Build history of the part. All positions in model axes, mm. A direction names the side the tool comes from. Round coordinates to 2 decimals unless told otherwise and drop trailing zeros. Write each loop counter-clockwise with the first axis right and the second up, starting at its lowest first coordinate (ties: lowest second). Pieces come first, ordered by that corner, then holes.
from build123d import *
from OCP.BRepFilletAPI import BRepFilletAPI_MakeChamfer

# Parameters (mm, degrees)
SKETCH1_W                = 15.2
SKETCH1_H                = 8.8
BOSS_EXTRUDE1_DEPTH      = 9
SKETCH3_W                = 13
SKETCH3_H                = 6.4
CUT_EXTRUDE1_DEPTH       = 8
SKETCH4_W                = 4.5
SKETCH4_H                = 1.2
CUT_EXTRUDE2_DEPTH       = 7
SKETCH5_W                = 3
SKETCH5_H                = 7
CUT_EXTRUDE3_DEPTH       = 1.1
SKETCH6_W                = 3
SKETCH6_H                = 7
CUT_EXTRUDE4_DEPTH       = 1.1
BOSS_EXTRUDE2_DEPTH      = 7.5
BOSS_EXTRUDE2_DEPTH_BACK = 4
SKETCH7_W                = 1
SKETCH7_H                = 1
CHAMFER1_SIZE            = 0.7
CHAMFER1_SIZE2           = 0.254779164
CHAMFER2_SIZE            = 0.5


with BuildPart() as part:
    # Sketch1 → Boss-Extrude1 (new body)
    with BuildSketch(Plane(origin=(0, 0, 0), x_dir=(1, 0, 0), z_dir=(0, 1, 0))):
        with Locations((7.6, 4.4)):
            Rectangle(SKETCH1_W, SKETCH1_H)
    extrude(amount=BOSS_EXTRUDE1_DEPTH)

    # Sketch3 → Cut-Extrude1 (cut)
    with BuildSketch(Plane(origin=(0, 9, 0), x_dir=(1, 0, 0), z_dir=(0, 1, 0))):
        with Locations((7.6, 4.4)):
            Rectangle(SKETCH3_W, SKETCH3_H)
    extrude(amount=-CUT_EXTRUDE1_DEPTH, mode=Mode.SUBTRACT)

    # Sketch4 → Cut-Extrude2 (cut)
    with BuildSketch(Plane(origin=(0, 9, 0), x_dir=(1, 0, 0), z_dir=(0, 1, 0))):
        with Locations((7.6, 0.6)):
            Rectangle(SKETCH4_W, SKETCH4_H)
    extrude(amount=-CUT_EXTRUDE2_DEPTH, mode=Mode.SUBTRACT)

    # Sketch5 → Cut-Extrude3 (cut)
    with BuildSketch(Plane.ZY):
        with Locations((-4.4, 3.5)):
            Rectangle(SKETCH5_W, SKETCH5_H)
    extrude(amount=-CUT_EXTRUDE3_DEPTH, mode=Mode.SUBTRACT)

    # Sketch6 → Cut-Extrude4 (cut)
    with BuildSketch(Plane(origin=(15.2, 0, 0), x_dir=(0, 0, -1), z_dir=(1, 0, 0))):
        with Locations((4.4, 3.5)):
            Rectangle(SKETCH6_W, SKETCH6_H)
    extrude(amount=-CUT_EXTRUDE4_DEPTH, mode=Mode.SUBTRACT)

    # Sketch7 → Boss-Extrude2 (add, two sides: drawn at the far end of the back side and taken through both)
    with BuildSketch(Plane(origin=(0, 1, 0), x_dir=(1, 0, 0), z_dir=(0, 1, 0)).offset(-BOSS_EXTRUDE2_DEPTH_BACK)):
        with Locations((7.6, 5.67)):
            Rectangle(SKETCH7_W, SKETCH7_H)
        with Locations((5.06, 5.67)):
            Rectangle(SKETCH7_W, SKETCH7_H)
        with Locations((10.14, 5.67)):
            Rectangle(SKETCH7_W, SKETCH7_H)
        with Locations((7.6, 3.13)):
            Rectangle(SKETCH7_W, SKETCH7_H)
        with Locations((10.14, 3.13)):
            Rectangle(SKETCH7_W, SKETCH7_H)
        with Locations((5.06, 3.13)):
            Rectangle(SKETCH7_W, SKETCH7_H)
    extrude(amount=BOSS_EXTRUDE2_DEPTH + BOSS_EXTRUDE2_DEPTH_BACK)

    # Chamfer1: one chamfer whose edges measure the first distance from different faces: ONE call of the kernel's chamfer builder (chamfer() names one face for all edges)
    chamfer1_edges_1 = [part.edges().sort_by_distance(p)[0] for p in [
        (7.1, 8.5, -5.67),
    ]]
    chamfer1_side_1 = [part.faces().sort_by_distance(p)[0] for p in [
        (7.1, 4.75, -5.67),
    ]]
    chamfer1_edges_2 = [part.edges().sort_by_distance(p)[0] for p in [
        (7.6, 8.5, -5.17),
    ]]
    chamfer1_side_2 = [part.faces().sort_by_distance(p)[0] for p in [
        (7.6, 4.75, -5.17),
    ]]
    chamfer1_edges_3 = [part.edges().sort_by_distance(p)[0] for p in [
        (8.1, 8.5, -5.67),
    ]]
    chamfer1_side_3 = [part.faces().sort_by_distance(p)[0] for p in [
        (8.1, 4.75, -5.67),
    ]]
    chamfer1_edges_4 = [part.edges().sort_by_distance(p)[0] for p in [
        (7.6, 8.5, -6.17),
    ]]
    chamfer1_side_4 = [part.faces().sort_by_distance(p)[0] for p in [
        (7.6, 4.75, -6.17),
    ]]
    chamfer1_edges_5 = [part.edges().sort_by_distance(p)[0] for p in [
        (9.64, 8.5, -5.67),
    ]]
    chamfer1_side_5 = [part.faces().sort_by_distance(p)[0] for p in [
        (9.64, 4.75, -5.67),
    ]]
    chamfer1_edges_6 = [part.edges().sort_by_distance(p)[0] for p in [
        (10.14, 8.5, -5.17),
    ]]
    chamfer1_side_6 = [part.faces().sort_by_distance(p)[0] for p in [
        (10.14, 4.75, -5.17),
    ]]
    chamfer1_edges_7 = [part.edges().sort_by_distance(p)[0] for p in [
        (10.64, 8.5, -5.67),
    ]]
    chamfer1_side_7 = [part.faces().sort_by_distance(p)[0] for p in [
        (10.64, 4.75, -5.67),
    ]]
    chamfer1_edges_8 = [part.edges().sort_by_distance(p)[0] for p in [
        (10.14, 8.5, -6.17),
    ]]
    chamfer1_side_8 = [part.faces().sort_by_distance(p)[0] for p in [
        (10.14, 4.75, -6.17),
    ]]
    chamfer1_edges_9 = [part.edges().sort_by_distance(p)[0] for p in [
        (7.1, 8.5, -3.13),
    ]]
    chamfer1_side_9 = [part.faces().sort_by_distance(p)[0] for p in [
        (7.1, 4.75, -3.13),
    ]]
    chamfer1_edges_10 = [part.edges().sort_by_distance(p)[0] for p in [
        (7.6, 8.5, -2.63),
    ]]
    chamfer1_side_10 = [part.faces().sort_by_distance(p)[0] for p in [
        (7.6, 4.75, -2.63),
    ]]
    chamfer1_edges_11 = [part.edges().sort_by_distance(p)[0] for p in [
        (8.1, 8.5, -3.13),
    ]]
    chamfer1_side_11 = [part.faces().sort_by_distance(p)[0] for p in [
        (8.1, 4.75, -3.13),
    ]]
    chamfer1_edges_12 = [part.edges().sort_by_distance(p)[0] for p in [
        (7.6, 8.5, -3.63),
    ]]
    chamfer1_side_12 = [part.faces().sort_by_distance(p)[0] for p in [
        (7.6, 4.75, -3.63),
    ]]
    chamfer1_edges_13 = [part.edges().sort_by_distance(p)[0] for p in [
        (9.64, 8.5, -3.13),
    ]]
    chamfer1_side_13 = [part.faces().sort_by_distance(p)[0] for p in [
        (9.64, 4.75, -3.13),
    ]]
    chamfer1_edges_14 = [part.edges().sort_by_distance(p)[0] for p in [
        (10.14, 8.5, -2.63),
    ]]
    chamfer1_side_14 = [part.faces().sort_by_distance(p)[0] for p in [
        (10.14, 4.75, -2.63),
    ]]
    chamfer1_edges_15 = [part.edges().sort_by_distance(p)[0] for p in [
        (10.64, 8.5, -3.13),
    ]]
    chamfer1_side_15 = [part.faces().sort_by_distance(p)[0] for p in [
        (10.64, 4.75, -3.13),
    ]]
    chamfer1_edges_16 = [part.edges().sort_by_distance(p)[0] for p in [
        (10.14, 8.5, -3.63),
    ]]
    chamfer1_side_16 = [part.faces().sort_by_distance(p)[0] for p in [
        (10.14, 4.75, -3.63),
    ]]
    chamfer1_edges_17 = [part.edges().sort_by_distance(p)[0] for p in [
        (4.56, 8.5, -3.13),
    ]]
    chamfer1_side_17 = [part.faces().sort_by_distance(p)[0] for p in [
        (4.56, 4.75, -3.13),
    ]]
    chamfer1_edges_18 = [part.edges().sort_by_distance(p)[0] for p in [
        (5.06, 8.5, -2.63),
    ]]
    chamfer1_side_18 = [part.faces().sort_by_distance(p)[0] for p in [
        (5.06, 4.75, -2.63),
    ]]
    chamfer1_edges_19 = [part.edges().sort_by_distance(p)[0] for p in [
        (5.56, 8.5, -3.13),
    ]]
    chamfer1_side_19 = [part.faces().sort_by_distance(p)[0] for p in [
        (5.56, 4.75, -3.13),
    ]]
    chamfer1_edges_20 = [part.edges().sort_by_distance(p)[0] for p in [
        (5.06, 8.5, -3.63),
    ]]
    chamfer1_side_20 = [part.faces().sort_by_distance(p)[0] for p in [
        (5.06, 4.75, -3.63),
    ]]
    chamfer1_edges_21 = [part.edges().sort_by_distance(p)[0] for p in [
        (4.56, 8.5, -5.67),
    ]]
    chamfer1_side_21 = [part.faces().sort_by_distance(p)[0] for p in [
        (4.56, 4.75, -5.67),
    ]]
    chamfer1_edges_22 = [part.edges().sort_by_distance(p)[0] for p in [
        (5.06, 8.5, -5.17),
    ]]
    chamfer1_side_22 = [part.faces().sort_by_distance(p)[0] for p in [
        (5.06, 4.75, -5.17),
    ]]
    chamfer1_edges_23 = [part.edges().sort_by_distance(p)[0] for p in [
        (5.56, 8.5, -5.67),
    ]]
    chamfer1_side_23 = [part.faces().sort_by_distance(p)[0] for p in [
        (5.56, 4.75, -5.67),
    ]]
    chamfer1_edges_24 = [part.edges().sort_by_distance(p)[0] for p in [
        (5.06, 8.5, -6.17),
    ]]
    chamfer1_side_24 = [part.faces().sort_by_distance(p)[0] for p in [
        (5.06, 4.75, -6.17),
    ]]
    chamfer1 = BRepFilletAPI_MakeChamfer(part.part.solid().wrapped)
    for e in chamfer1_edges_1:
        chamfer1.Add(CHAMFER1_SIZE, CHAMFER1_SIZE2, e.wrapped, chamfer1_side_1[0].wrapped)  # the first distance lies on this face
    for e in chamfer1_edges_2:
        chamfer1.Add(CHAMFER1_SIZE, CHAMFER1_SIZE2, e.wrapped, chamfer1_side_2[0].wrapped)  # the first distance lies on this face
    for e in chamfer1_edges_3:
        chamfer1.Add(CHAMFER1_SIZE, CHAMFER1_SIZE2, e.wrapped, chamfer1_side_3[0].wrapped)  # the first distance lies on this face
    for e in chamfer1_edges_4:
        chamfer1.Add(CHAMFER1_SIZE, CHAMFER1_SIZE2, e.wrapped, chamfer1_side_4[0].wrapped)  # the first distance lies on this face
    for e in chamfer1_edges_5:
        chamfer1.Add(CHAMFER1_SIZE, CHAMFER1_SIZE2, e.wrapped, chamfer1_side_5[0].wrapped)  # the first distance lies on this face
    for e in chamfer1_edges_6:
        chamfer1.Add(CHAMFER1_SIZE, CHAMFER1_SIZE2, e.wrapped, chamfer1_side_6[0].wrapped)  # the first distance lies on this face
    for e in chamfer1_edges_7:
        chamfer1.Add(CHAMFER1_SIZE, CHAMFER1_SIZE2, e.wrapped, chamfer1_side_7[0].wrapped)  # the first distance lies on this face
    for e in chamfer1_edges_8:
        chamfer1.Add(CHAMFER1_SIZE, CHAMFER1_SIZE2, e.wrapped, chamfer1_side_8[0].wrapped)  # the first distance lies on this face
    for e in chamfer1_edges_9:
        chamfer1.Add(CHAMFER1_SIZE, CHAMFER1_SIZE2, e.wrapped, chamfer1_side_9[0].wrapped)  # the first distance lies on this face
    for e in chamfer1_edges_10:
        chamfer1.Add(CHAMFER1_SIZE, CHAMFER1_SIZE2, e.wrapped, chamfer1_side_10[0].wrapped)  # the first distance lies on this face
    for e in chamfer1_edges_11:
        chamfer1.Add(CHAMFER1_SIZE, CHAMFER1_SIZE2, e.wrapped, chamfer1_side_11[0].wrapped)  # the first distance lies on this face
    for e in chamfer1_edges_12:
        chamfer1.Add(CHAMFER1_SIZE, CHAMFER1_SIZE2, e.wrapped, chamfer1_side_12[0].wrapped)  # the first distance lies on this face
    for e in chamfer1_edges_13:
        chamfer1.Add(CHAMFER1_SIZE, CHAMFER1_SIZE2, e.wrapped, chamfer1_side_13[0].wrapped)  # the first distance lies on this face
    for e in chamfer1_edges_14:
        chamfer1.Add(CHAMFER1_SIZE, CHAMFER1_SIZE2, e.wrapped, chamfer1_side_14[0].wrapped)  # the first distance lies on this face
    for e in chamfer1_edges_15:
        chamfer1.Add(CHAMFER1_SIZE, CHAMFER1_SIZE2, e.wrapped, chamfer1_side_15[0].wrapped)  # the first distance lies on this face
    for e in chamfer1_edges_16:
        chamfer1.Add(CHAMFER1_SIZE, CHAMFER1_SIZE2, e.wrapped, chamfer1_side_16[0].wrapped)  # the first distance lies on this face
    for e in chamfer1_edges_17:
        chamfer1.Add(CHAMFER1_SIZE, CHAMFER1_SIZE2, e.wrapped, chamfer1_side_17[0].wrapped)  # the first distance lies on this face
    for e in chamfer1_edges_18:
        chamfer1.Add(CHAMFER1_SIZE, CHAMFER1_SIZE2, e.wrapped, chamfer1_side_18[0].wrapped)  # the first distance lies on this face
    for e in chamfer1_edges_19:
        chamfer1.Add(CHAMFER1_SIZE, CHAMFER1_SIZE2, e.wrapped, chamfer1_side_19[0].wrapped)  # the first distance lies on this face
    for e in chamfer1_edges_20:
        chamfer1.Add(CHAMFER1_SIZE, CHAMFER1_SIZE2, e.wrapped, chamfer1_side_20[0].wrapped)  # the first distance lies on this face
    for e in chamfer1_edges_21:
        chamfer1.Add(CHAMFER1_SIZE, CHAMFER1_SIZE2, e.wrapped, chamfer1_side_21[0].wrapped)  # the first distance lies on this face
    for e in chamfer1_edges_22:
        chamfer1.Add(CHAMFER1_SIZE, CHAMFER1_SIZE2, e.wrapped, chamfer1_side_22[0].wrapped)  # the first distance lies on this face
    for e in chamfer1_edges_23:
        chamfer1.Add(CHAMFER1_SIZE, CHAMFER1_SIZE2, e.wrapped, chamfer1_side_23[0].wrapped)  # the first distance lies on this face
    for e in chamfer1_edges_24:
        chamfer1.Add(CHAMFER1_SIZE, CHAMFER1_SIZE2, e.wrapped, chamfer1_side_24[0].wrapped)  # the first distance lies on this face
    add(Compound.cast(chamfer1.Shape()), mode=Mode.REPLACE)

    # Chamfer2
    chamfer2_edges = [part.edges().sort_by_distance(p)[0] for p in [
        (1.1, 9, -4.4),
        (3.225, 9, -1.2),
        (14.1, 9, -4.4),
        (7.6, 9, -7.6),
        (11.975, 9, -1.2),
    ]]
    chamfer(chamfer2_edges, length=CHAMFER2_SIZE)


solid = part.part
1) Pin check, flat tips, straight feed: pin 1 Ø1.1 at (x, y) = (5, -2) entering from -Z; pin 2 Ø1.1 at (y, z) = (-2, -5.5) entering from +X; pin 3 Ø0.5 at (y, z) = (3, -5.5) entering from -X. Stop position of each tip, or through.
Results:
pin 1: stops at z = -6.17
pin 2: stops at x = 10.64
pin 3: stops at x = 4.56
2) Which spindle directions (+Z, -Z, +X, -X, +Y, -Y) get a long thin tool onto all of the face, cutting with end or side? Do faces 4 (the flat face through (5.35, 6, -1)), 5 (the flat face through (0.5, 7, -4.4)), 6 (the flat face through (10.64, -2, -6)). Say none if no direction does.
Results:
face 4: +Z, +Y
face 5: -X, -Y
face 6: +Z, -Z, +X, -Y
3) Slice it at D-D (z = -7). Write the cut outline in (x, y).
Results:
outline: (0, 0) - (15.2, 0) - (15.2, 9) - (14.6, 9) - (14.1, 8.5) - (14.1, 1) - (1.1, 1) - (1.1, 8.5) - (0.6, 9) - (0, 9) - close
4) Slice it at A-A (y = -0.25). Write the cut outline in (x, z).
Results:
outline: (4.56, -6.17) - (5.56, -6.17) - (5.56, -5.17) - (4.56, -5.17) - close; (4.56, -3.63) - (5.56, -3.63) - (5.56, -2.63) - (4.56, -2.63) - close; (7.1, -6.17) - (8.1, -6.17) - (8.1, -5.17) - (7.1, -5.17) - close; (7.1, -3.63) - (8.1, -3.63) - (8.1, -2.63) - (7.1, -2.63) - close; (9.64, -6.17) - (10.64, -6.17) - (10.64, -5.17) - (9.64, -5.17) - close; (9.64, -3.63) - (10.64, -3.63) - (10.64, -2.63) - (9.64, -2.63) - close
5) Wall check: L1, parallel to Z at x = 10.25, y = 7.5; L2, parallel to X at y = 6.75, z = -3; L3, parallel to Z at x = 5.5, y = 3.25. Give the ranges that are in metal, low to high.
Results:
L1: z = -8.8 to -7.6, -6.17 to -5.17, -3.63 to -2.63, -1.2 to 0
L2: x = 4.56 to 5.56, 7.1 to 8.1, 9.64 to 10.64
L3: z = -8.8 to -7.6, -6.17 to -5.17, -3.63 to -2.63
6) Mould opens along Z. For faces 1 (the flat face through (15.2, 4.4, -6.3)), 2 (the flat face through (5, -2, -2.63)), 3 (the flat face through (10, 4, -5.17)) say: released by +Z, released by -Z, zero draft, split by the parting line, or undercut.
Results:
face 1: zero draft
face 2: released by +Z
face 3: undercut
7) Slice it at C-C (x = 3). Write the cut outline in (y, z), plus the area to 4 significant figures.
Results:
outline: (0, -8.8) - (9, -8.8) - (9, -8.1) - (8.5, -7.6) - (1, -7.6) - (1, -1.2) - (8.5, -1.2) - (9, -0.7) - (9, 0) - (0, 0) - close
area: 27.75 mm2
8) Slice it at B-B (z = -4.25). Write the cut outline in (x, y).
Results:
outline: (0, 7) - (1.1, 7) - (1.1, 8.5) - (0.6, 9) - (0, 9) - close; (1.1, 0) - (14.1, 0) - (14.1, 1) - (1.1, 1) - close; (14.1, 7) - (15.2, 7) - (15.2, 9) - (14.6, 9) - (14.1, 8.5) - close
